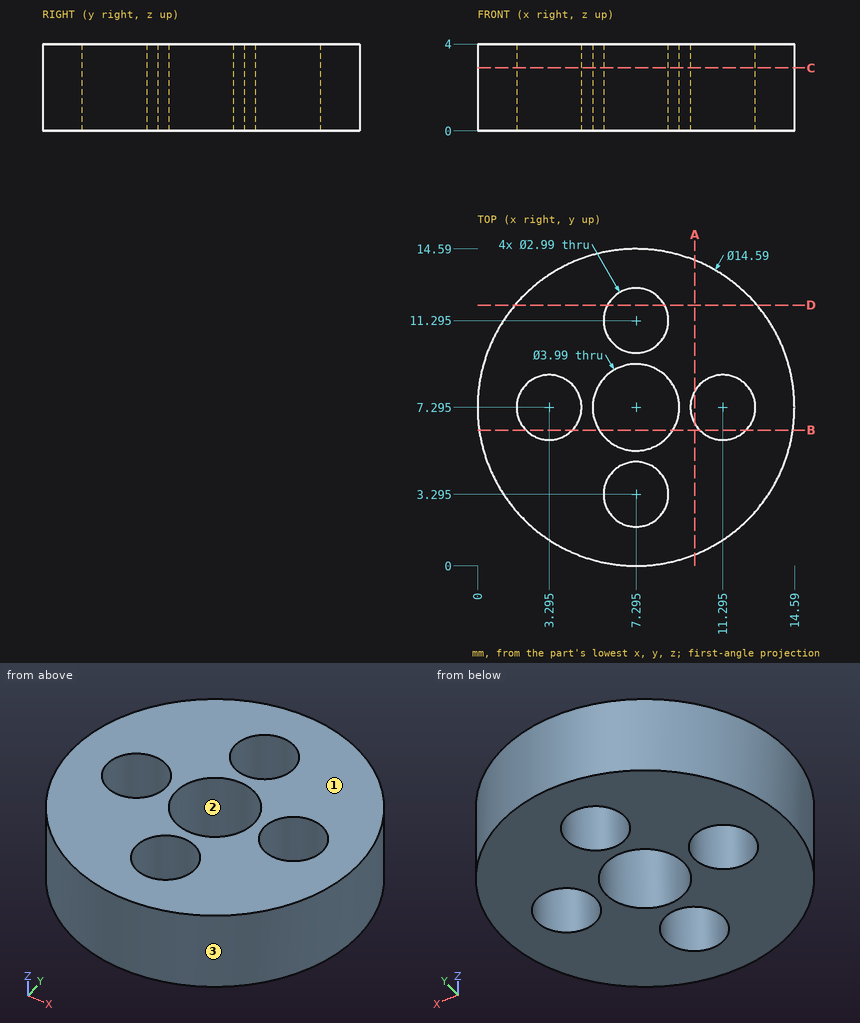
The figure shows three views and two pictorial views of one solid part (mm, origin at its lowest corner). Answer the questions. Give positions to 0.01 mm unless a question says otherwise; leave off trailing zeros. Loops run counter-clockwise (first coordinate to the right, second up) from the corner with the lowest first, then second, coordinate; pieces in that order, holes last. Notation, with made-up numbers: (55.25, 7.25) -> (59.25, 7.25) arc R25 ccw to (59.25, 36.25) -> close; hole circle Ø11 at (16, 10). An arc over 180 degrees is marked (long way). Use a Markdown table: item, result. Add a question column.
1. Section D-D on y = 12 is taken. Determine the outline of the cut face in (x, z), and give its area (3 significant figures).
2. Determine the mould class of the marked faces 1, 2 and 3 for opening direction X: released by +X, released by -X, zero draft, split by the parting line, or undercut.
3. Section A-A on x = 10 is taken. Determine the outline of the cut face in (y, z), and give its area (3 significant figures).
4. Section B-B on y = 6.25 is taken. Determine the outline of the cut face in (x, z).
5. Section C-C on z = 2.9 is taken. Determine the outline of the cut face in (x, y) (3 decimals).
6. Find the intervals of material crossed by probe 1 along X at (y, z) = (7.25, 2.15); probe 2 along Y at (x, z) = (7, 1.6); probe 3 along Y at (x, z) = (7.75, 2.35), in increasing order.
7. Flat-ended cylindrical pins translate along their axes: pin 1 Ø2.5 at (x, y) = (7.295, 7.295) entering from +Z; pin 2 Ø1 at (x, z) = (6.5, 2) entering from -Y. Find the tip coordinate at first contact, or state that the pin passes through.
Results below:
| question | item | result |
|---|---|---|
| 1 | outline | (1.72, 0) -> (5.98, 0) -> (5.98, 4) -> (1.72, 4) -> close; (8.61, 0) -> (12.87, 0) -> (12.87, 4) -> (8.61, 4) -> close |
| 1 | area | 34.1 mm^2 |
| 2 | face 1 | zero draft |
| 2 | face 2 | undercut |
| 2 | face 3 | split by the parting line |
| 3 | outline | (0.52, 0) -> (6.55, 0) -> (6.55, 4) -> (0.52, 4) -> close; (8.04, 0) -> (14.07, 0) -> (14.07, 4) -> (8.04, 4) -> close |
| 3 | area | 48.2 mm^2 |
| 4 | outline | (0.08, 0) -> (2.23, 0) -> (2.23, 4) -> (0.08, 4) -> close; (4.36, 0) -> (5.6, 0) -> (5.6, 4) -> (4.36, 4) -> close; (8.99, 0) -> (10.23, 0) -> (10.23, 4) -> (8.99, 4) -> close; (12.36, 0) -> (14.51, 0) -> (14.51, 4) -> (12.36, 4) -> close |
| 5 | outline | circle Ø14.59 at (7.295, 7.295); hole circle Ø2.99 at (3.295, 7.295); hole circle Ø3.99 at (7.295, 7.295); hole circle Ø2.99 at (7.295, 3.295); hole circle Ø2.99 at (7.295, 11.295); hole circle Ø2.99 at (11.295, 7.295) |
| 6 | probe 1 | x = 0 to 1.8, 4.79 to 5.3, 9.29 to 9.8, 12.79 to 14.59 |
| 6 | probe 2 | y = 0.01 to 1.83, 4.76 to 5.32, 9.27 to 9.83, 12.76 to 14.58 |
| 6 | probe 3 | y = 0.01 to 1.87, 4.72 to 5.35, 9.24 to 9.87, 12.72 to 14.58 |
| 7 | pin 1 | passes through |
| 7 | pin 2 | stops at y = 0.01 |
